Geometry: see drawing. Coordinates: mm, zero at the bounding-box minimum. Coordinates: 2 decimals unless noted, no trailing zeros. Write each loop counter-clockwise with the first axis right and the second up, starting at its lowest first coordinate (ties: lowest second). Pieces come first, ordered by that corner, then holes. Notation, with made-up numbers: M 78.25,1 L 120.25,1 A30 ccw 120.25,24 Z; hole C -30.5,73 d2. An arc over 180 degrees is marked long. Write item = value, one per line. Start each with the question number.
1. Pin query (flat end, axial travel): pin 1 Ø6 at (x, z) = (5, 115) entering from +Y. Return the tip coordinate at first contact, or that it passes through.
2. Section query B-B (z = 115). Output: boundary loops of the cut face in (x, y).
3. Line query: line 1 along Z through (x, y) = (5, 0.95); line 2 along Z through (x, y) = (59.5, 1.35); line 3 along X through (y, z) = (0.5, 115). Output: solid intervals per line, ascending.
4. Section query A-A (x = 60). Output: boundary loops of the cut face in (y, z).
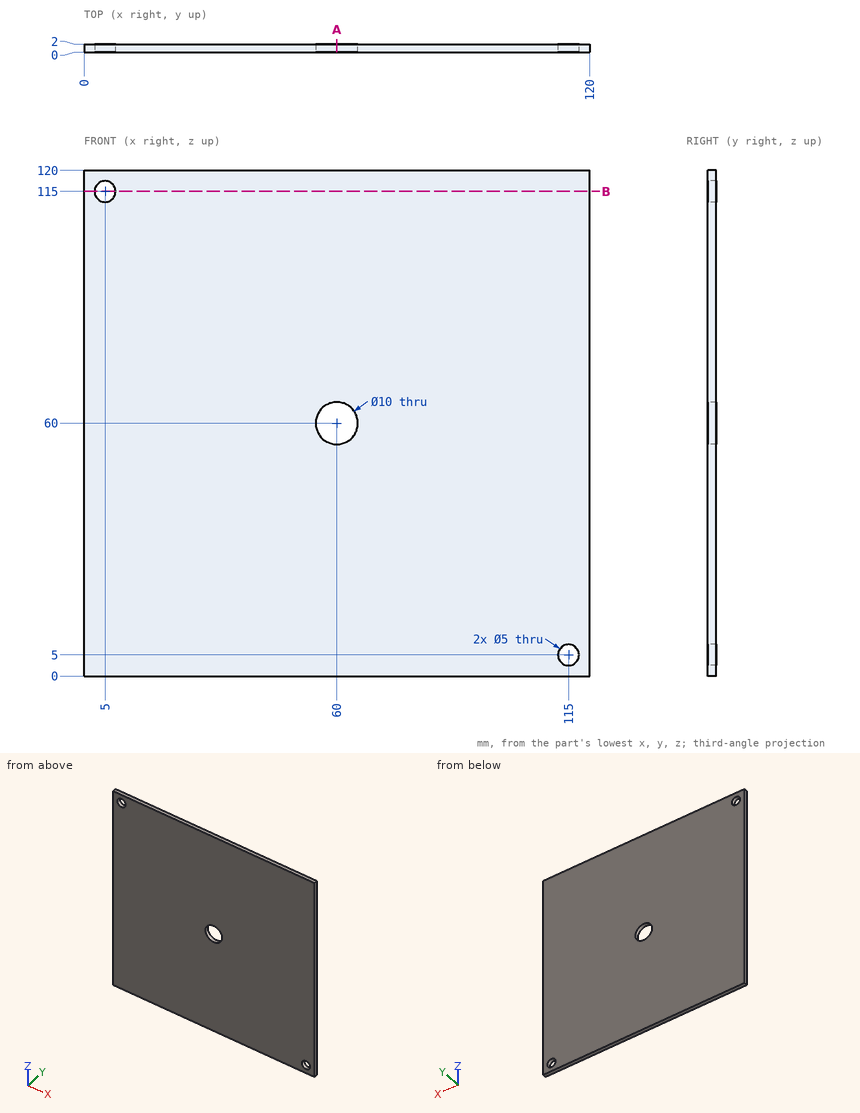
Results are:
q1.pin_1 = 2
q2.outline = M 0,0 L 2.5,0 L 2.5,2 L 0,2 Z; M 7.5,0 L 120,0 L 120,2 L 7.5,2 Z
q3.line_1 = 0 to 112.5, 117.5 to 120
q3.line_2 = 0 to 55.03, 64.97 to 120
q3.line_3 = 0 to 2.5, 7.5 to 120
q4.outline = M 0,0 L 2,0 L 2,55 L 0,55 Z; M 0,65 L 2,65 L 2,120 L 0,120 Z
